Design review of the part built by this model. Coordinates are the model's own, in mm. A direction names the side the tool comes from. Coordinates: 2 decimals unless noted, no trailing zeros. Loops run counter-clockwise (first coordinate to the right, second up) from the corner with the lowest first, then second, coordinate; pieces in that order, holes last. Notation, with made-up numbers: M 74.5,75.25 L 125.5,75.25 A16 cw 125.5,95.25 Z; hole C 62.5,84 d11. An arc over 180 degrees is marked long. Put each result on its own line as item: value. Start each with the question number.
(1) For probe 1 along X at (y, z) = (2.5, 7.25); probe 2 along Z at (x, y) = (25, 7.75); probe 3 along Y at (x, z) = (15, 13.7), list the stretches that pass through material, from the lowest coordinate up. Write a range as [from, to].
(2) Take a section at B-B, the plane y = 5. Give the boundary of the cut face in (x, z), then the cut area to 3 significant figures.
(3) Take a section at C-C, the plane z = 8.75. Give the boundary of the cut face in (x, y), then the cut area to 3 significant figures.
(4) For faces 1 (the cylindrical face through (17.494, 3.966, 12.288)), 2 (the flat face through (18.363, 5, 7)), list the 3-axis set-ups (+Z, -Z, +X, -X, +Y, -Y) from which the entire face can be reached by the end or side of a thin tool; tool diameter is ignored.
(5) Take a section at D-D, the plane x = 5. Give the boundary of the cut face in (y, z).
(6) Take a section at A-A, the plane x = 15. Give the boundary of the cut face in (y, z), then the cut area to 3 significant figures.
(7) Clearance check with a flat-ended pin moving along its axis: pin 1 (7 mm diameter, centred on x = 5, z = 5, fed in from +Y). State where the tip first meets the part, or that it passes through.
(8) The part is to be moulded in two halves that separate along Z. For faces 3 (the flat face through (0, 5, 7)), 4 (the cylindrical face through (4.415, 4.93, 2.364)), 5 (the flat face through (12, 4, 9.5)), 6 (the flat face through (11, 5, 15)), say which applies: +Z half, -Z half, draft (parallel to the pull), parting line (faces both ways), or undercut.
```python
from build123d import *

# Parameters (mm, degrees)
SKETCH_AS_DRAWN_W              = 30
SKETCH_AS_DRAWN_H              = 15
SKETCH_AS_DRAWN_R              = 2.7
EXTRUDE_DEPTH                  = 10
EXTRUDE_ONTO_SKETCH_ROLL_ANGLE = 90
SKETCH001_R                    = 2.7
POCKET_DEPTH                   = 15.001
SKETCH002_W                    = 8.2
SKETCH002_H                    = 4.5
POCKET001_DEPTH                = 10.001


with BuildPart() as part:
    # Sketch as drawn → Extrude (new)
    with BuildSketch(Plane.XY):
        with Locations((15, 7.5)):
            Rectangle(SKETCH_AS_DRAWN_W, SKETCH_AS_DRAWN_H)
        with Locations((5, 5)):
            Circle(SKETCH_AS_DRAWN_R, mode=Mode.SUBTRACT)
        with Locations((25, 5)):
            Circle(SKETCH_AS_DRAWN_R, mode=Mode.SUBTRACT)
    extrude(amount=-EXTRUDE_DEPTH)


with BuildPart() as part_1:
    # Extrude onto Sketch roll: moved
    add(part.part.rotate(Axis((0, 0, 0), (1, 0, 0)), EXTRUDE_ONTO_SKETCH_ROLL_ANGLE))


with BuildPart() as part_2:
    # Extrude onto Sketch placement: moved
    add(part_1.part)

    # Sketch001 → Pocket (cut, through all)
    with BuildSketch(Plane.XY.offset(15)):
        with Locations((15, 5)):
            Circle(SKETCH001_R)
    extrude(amount=-POCKET_DEPTH, mode=Mode.SUBTRACT)

    # Sketch002 → Pocket001 (cut, through all)
    with BuildSketch(Plane.XZ):
        with Locations((14.263317, 7.25)):
            Rectangle(SKETCH002_W, SKETCH002_H)
    extrude(amount=-POCKET001_DEPTH, mode=Mode.SUBTRACT)


solid = part_2.part
```
Computed values:
1. probe 1: x = [0, 3.51], [6.49, 10.16], [18.36, 23.51], [26.49, 30]
1. probe 2: z = [0, 2.3], [7.7, 15]
1. probe 3: y = [0, 2.3], [7.7, 10]
2. outline: M 0,0 L 12.3,0 L 12.3,5 L 10.16,5 L 10.16,9.5 L 12.3,9.5 L 12.3,15 L 0,15 Z; M 17.7,0 L 30,0 L 30,15 L 17.7,15 L 17.7,9.5 L 18.36,9.5 L 18.36,5 L 17.7,5 Z; hole C 5,5 d5.4; hole C 25,5 d5.4
2. area: 311 mm^2
3. outline: M 0,0 L 10.16,0 L 10.16,10 L 0,10 Z; M 18.36,0 L 30,0 L 30,10 L 18.36,10 Z
3. area: 218 mm^2
4. face 1: +Z, -Z
4. face 2: +Y, -Y
5. outline: M 0,0 L 10,0 L 10,2.3 L 0,2.3 Z; M 0,7.7 L 10,7.7 L 10,15 L 0,15 Z
6. outline: M 0,0 L 2.3,0 L 2.3,5 L 0,5 Z; M 0,9.5 L 2.3,9.5 L 2.3,15 L 0,15 Z; M 7.7,0 L 10,0 L 10,5 L 7.7,5 Z; M 7.7,9.5 L 10,9.5 L 10,15 L 7.7,15 Z
6. area: 48.3 mm^2
7. pin 1: stops at y = 10
8. face 3: draft
8. face 4: undercut
8. face 5: undercut
8. face 6: +Z half
